from build123d import *

# Parameters (mm, degrees)
F0_W     = 101.6
F0_H     = 50.8
F1_DEPTH = 76.2
F2_R     = 6.35
F3_DEPTH = 76.201
F4_W     = 25.4
F4_H     = 38.1
F6_W     = 6.35
F6_H     = 12.7


with BuildPart() as f1:
    # F0 (on Front) → F1 (new body)
    with BuildSketch(Plane.XZ):
        Rectangle(F0_W, F0_H)
    extrude(amount=-F1_DEPTH)

    # F2 (on face) → F3 (cut, through all)
    with BuildSketch(Plane.XZ):
        with Locations((-38.1, 12.7)):
            Circle(F2_R)
        with Locations((-38.1, -12.7)):
            Circle(F2_R)
        with Locations((38.1, -12.7)):
            Circle(F2_R)
        with Locations((38.1, 12.7)):
            Circle(F2_R)
    extrude(amount=-F3_DEPTH, mode=Mode.SUBTRACT)

    # F4 (on Top) → F5 (revolve)
    with BuildSketch(Plane.XY):
        with Locations((12.7, 95.25)):
            Rectangle(F4_W, F4_H)
    revolve(axis=Axis((0, 95.25, 0), (0, 1, 0)))

    # F6 (on Top) → F7 (revolve, cut)
    with BuildSketch(Plane.XY):
        with Locations((22.225, 95.25)):
            Rectangle(F6_W, F6_H)
    revolve(axis=Axis((0, 70.217416, 0), (0, 1, 0)), mode=Mode.SUBTRACT)


solid = f1.part
Can you work these out from the model? Positions are in its coordinate system, mm. A direction names the side the tool comes from. Coordinates: 2 decimals unless noted, no trailing zeros. Order: outer loops, then holes, each group sorted by start corner. A loop starts at its lowest first (then second) coordinate and runs counter-clockwise, first axis right, second up. Notation, with made-up numbers: (-18.75, -16) -> (22.25, -16) arc R12 cw to (22.25, -11) -> close; hole circle Ø11 at (85.25, -35.75). An arc over 180 degrees is marked (long way). Use one line per item in the form item = value.
Q1. Which directions (+Z, -Z, +X, -X, +Y, -Y) give clear straight access to the entire face, cutting with the end or side of a thin tool? Please do faces 5 (the face through (-15.12, 95.34, 11.59)), 6 (the face through (31, 76.2, 0)), 7 (the face through (31.756, 37.567, -12.421)), 8 (the face through (-5.506, 82.639, 24.796)).
From the geometry:
face_5 = none
face_6 = +X, +Y
face_7 = +Y, -Y
face_8 = +Y
Q2. Imagine slicing it at B-B, the plane y = 59. List the corners of the cut face in (x, z) for me, then the cut area to 3 significant figures.
From the geometry:
outline = (-50.8, -25.4) -> (50.8, -25.4) -> (50.8, 25.4) -> (-50.8, 25.4) -> close; hole circle Ø12.7 at (-38.1, -12.7); hole circle Ø12.7 at (-38.1, 12.7); hole circle Ø12.7 at (38.1, -12.7); hole circle Ø12.7 at (38.1, 12.7)
area = 4,650 mm²
Q3. We'd pull the mould along Z, two halves only. Please class faces 1 (the face through (0, 114.3, 0)), 2 (the face through (-1, 38, 25.4)), 3 (the face through (-5.506, 108.039, 24.796)), 4 (the face through (-32.234, 37.567, -15.132)): released by +Z, released by -Z, zero draft, split by the parting line, or undercut.
From the geometry:
face_1 = zero draft
face_2 = released by +Z
face_3 = split by the parting line
face_4 = undercut
Q4. Imagine slicing it at D-D, the plane z = 12.7. List the corners of the cut face in (x, y) for me, then the cut area to 3 significant figures.
From the geometry:
outline = (-50.8, 0) -> (-44.45, 0) -> (-44.45, 76.2) -> (-50.8, 76.2) -> close; (-31.75, 0) -> (31.75, 0) -> (31.75, 76.2) -> (22, 76.2) -> (22, 88.9) -> (14.2, 88.9) -> (14.2, 101.6) -> (22, 101.6) -> (22, 114.3) -> (-22, 114.3) -> (-22, 101.6) -> (-14.2, 101.6) -> (-14.2, 88.9) -> (-22, 88.9) -> (-22, 76.2) -> (-31.75, 76.2) -> close; (44.45, 0) -> (50.8, 0) -> (50.8, 76.2) -> (44.45, 76.2) -> close
area = 7,280 mm²
Q5. Will these pins go through, and if not, where does the flat tip stop? P1, Ø10, axis at x = 38.1, z = 12.7, coming from the +Y side; P2, Ø20.5, axis at x = 38.1, z = -12.7, coming from the +Y side.
From the geometry:
P1 = through
P2 = 76.2
Q6. Imagine slicing it at A-A, the plane x = -38.1. List the corners of the cut face in (y, z) for me, then the cut area to 3 significant figures.
From the geometry:
outline = (0, -25.4) -> (76.2, -25.4) -> (76.2, -19.05) -> (0, -19.05) -> close; (0, -6.35) -> (76.2, -6.35) -> (76.2, 6.35) -> (0, 6.35) -> close; (0, 19.05) -> (76.2, 19.05) -> (76.2, 25.4) -> (0, 25.4) -> close
area = 1,940 mm²
Q7. I need wall thicknesses on L1, parallel to Y at x = 18.5, z = 14.5; L2, parallel to X at y = 42.5, z = 7; L3, parallel to Z at x = -38.1, y = 16. Which ranges of each line are inside material? Lowest first, please.
From the geometry:
L1 = 0 to 88.9, 101.6 to 114.3
L2 = -50.8 to -40.9, -35.3 to 35.3, 40.9 to 50.8
L3 = -25.4 to -19.05, -6.35 to 6.35, 19.05 to 25.4
Q8. Imagine slicing it at C-C, the plane z = 0. List the corners of the cut face in (x, y) for me, then the cut area to 3 significant figures.
From the geometry:
outline = (-50.8, 0) -> (50.8, 0) -> (50.8, 76.2) -> (25.4, 76.2) -> (25.4, 88.9) -> (19.05, 88.9) -> (19.05, 101.6) -> (25.4, 101.6) -> (25.4, 114.3) -> (-25.4, 114.3) -> (-25.4, 101.6) -> (-19.05, 101.6) -> (-19.05, 88.9) -> (-25.4, 88.9) -> (-25.4, 76.2) -> (-50.8, 76.2) -> close
area = 9,520 mm²
